Build history of the part. All positions in model axes, mm. Face numbers are marked on the shaded views. A direction names the side the tool comes from. Round coordinates to 2 decimals unless told otherwise and drop trailing zeros. Order: outer loops, then holes, each group sorted by start corner. A loop starts at its lowest first (then second) coordinate and runs counter-clockwise, first axis right, second up. Notation, with made-up numbers: (-34, 12) -> (-22, 12) arc R14 cw to (-22, 18) -> close; hole circle Ø3 at (21.5, -39.5). An arc over 180 degrees is marked (long way). Answer as a JSON object with one key per item and string values.
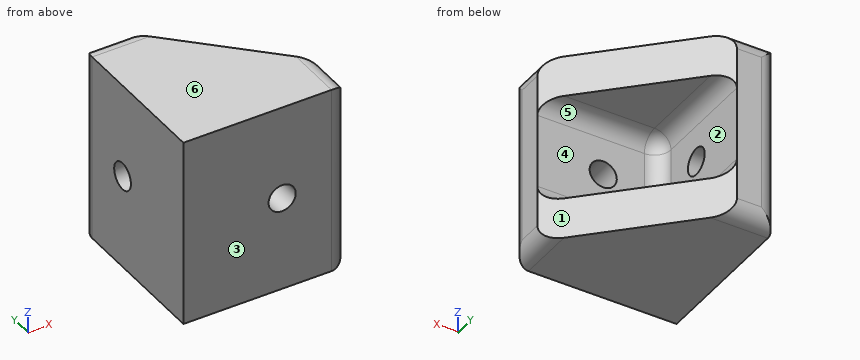
from build123d import *

# Parameters (mm, degrees)
BOSS_EXTRUDE2_DEPTH                   = 23
SHELL1_START                          = 5
SHELL1_OUTLINE_W                      = 16
SHELL1_OUTLINE_H                      = 13
SHELL1_DEPTH                          = 15
FILLET1_R                             = 2
FILLET3_R                             = 2
TAP_DRILL_FOR_M4X0_7_TAP1_D           = 3.3
TAP_DRILL_FOR_M4X0_7_TAP1_ON_FACE_2_D = 3.3


# Read off the part's stored shape, not the designer's step: Shell1
with BuildPart() as part:
    # Sketch1 → Boss-Extrude2 (new body)
    with BuildSketch(Plane.XY):
        Polygon((0, 0), (0, 20), (5, 20), (20, 5), (20, 0), align=None)
    extrude(amount=-BOSS_EXTRUDE2_DEPTH)

    # Shell1 outline → Shell1 (cut)
    with BuildSketch(Plane(origin=(0, 0, 0), x_dir=(1, 0, 0), z_dir=(0, 1, 0)).offset(SHELL1_START)):
        with Locations((13, 11.5)):
            Rectangle(SHELL1_OUTLINE_W, SHELL1_OUTLINE_H)
    extrude(amount=SHELL1_DEPTH, mode=Mode.SUBTRACT)

    # Fillet1
    fillet1_edges = [part.edges().sort_by_distance(p)[0] for p in [
        (12.5, 5, -18),
        (5, 12.5, -18),
        (5, 5, -11.5),
        (12.5, 5, -5),
        (5, 12.5, -5),
    ]]
    fillet(fillet1_edges, radius=FILLET1_R)

    # Fillet3
    fillet3_edges = [part.edges().sort_by_distance(p)[0] for p in [
        (2.5, 20, -23),
        (2.5, 20, 0),
        (20, 2.5, 0),
        (20, 2.5, -23),
        (0, 20, -11.5),
        (20, 0, -11.5),
    ]]
    fillet(fillet3_edges, radius=FILLET3_R)

    # Tap Drill for M4x0.7 Tap1 (through all)
    with Locations(Plane(origin=(5, 12, -11.5), x_dir=(0, 0, 1), z_dir=(1, 0, 0))):
        with Locations((0, 0)):
            Hole(TAP_DRILL_FOR_M4X0_7_TAP1_D / 2)

    # Tap Drill for M4x0.7 Tap1 on face 2 (through all)
    with Locations(Plane(origin=(12, 5, -11.5), x_dir=(0, 0, 1), z_dir=(0, 1, 0))):
        with Locations((0, 0)):
            Hole(TAP_DRILL_FOR_M4X0_7_TAP1_ON_FACE_2_D / 2)


solid = part.part
1) Cut at B-B, the plane x = 12. Give the cut face in (y, z), plus the area to 3 significant figures.
Checked values:
{"outline": "(0, -23) -> (13, -23) -> (13, -18) -> (7, -18) arc R2 cw to (5, -16) -> (5, -13.15) -> (0, -13.15) -> close; (0, -9.85) -> (5, -9.85) -> (5, -7) arc R2 cw to (7, -5) -> (13, -5) -> (13, 0) -> (0, 0) -> close", "area": "180 mm²"}
2) Cut at A-A, the plane z = -11.5. Give the cut face in (x, y), plus the area to 3 significant figures.
Checked values:
{"outline": "(0, 0) -> (10.35, 0) -> (10.35, 5) -> (7, 5) arc R2 cw to (5, 7) -> (5, 10.35) -> (0, 10.35) -> close; (0, 13.65) -> (5, 13.65) -> (5, 20) -> (2, 20) arc R2 ccw to (0, 18) -> close; (13.65, 0) -> (18, 0) arc R2 ccw to (20, 2) -> (20, 5) -> (13.65, 5) -> close", "area": "141 mm²"}
3) Cut at D-D, the plane z = -8. Give the cut face in (x, y).
Checked values:
{"outline": "(0, 0) -> (18, 0) arc R2 ccw to (20, 2) -> (20, 5) -> (7, 5) arc R2 cw to (5, 7) -> (5, 20) -> (2, 20) arc R2 ccw to (0, 18) -> close"}
4) Pull direction Z, two halves, no side cores. Call the marked faces 3, 4, 5 and 6: pulls with the +Z half, pulls with the -Z half, needs draft (parallel to the pull), parting line crosses it, or undercut.
Checked values:
{"face 3": "needs draft", "face 4": "undercut", "face 5": "undercut", "face 6": "pulls with the +Z half"}
5) Which spindle directions (+Z, -Z, +X, -X, +Y, -Y) get a long thin tool onto all of the face, cutting with end or side? Do the marked faces 1 and 2. Say none if no direction does.
Checked values:
{"face 1": "+Z, -Z, +X, +Y", "face 2": "+X, +Y"}
6) Probe L1, parallel to Y at x = 3.2, z = -11.5; L2, parallel to Z at x = 8.75, y = 14.5; L3, parallel to X at y = 14, z = -14.75. List the from-to ranges inside material, lowest first. Write a range as from..to.
Checked values:
{"L1": "y = 0..10.35, 13.65..20", "L2": "z = -23..-18, -5..0", "L3": "x = 0..5"}
7) Flat gauge pins, fed straight in: pin 1 Ø4.5 at (y, z) = (10.5, -12) entering from +X; pin 2 Ø3 at (y, z) = (12, -11.5) entering from +X; pin 3 Ø2.5 at (x, z) = (13.5, -10.5) entering from +Y; pin 4 Ø1.5 at (y, z) = (15.5, -16.5) entering from +X. Where does each tip first touch, or does it go through?
Checked values:
{"pin 1": "stops at x = 5", "pin 2": "passes through", "pin 3": "stops at y = 5", "pin 4": "stops at x = 5.44"}
